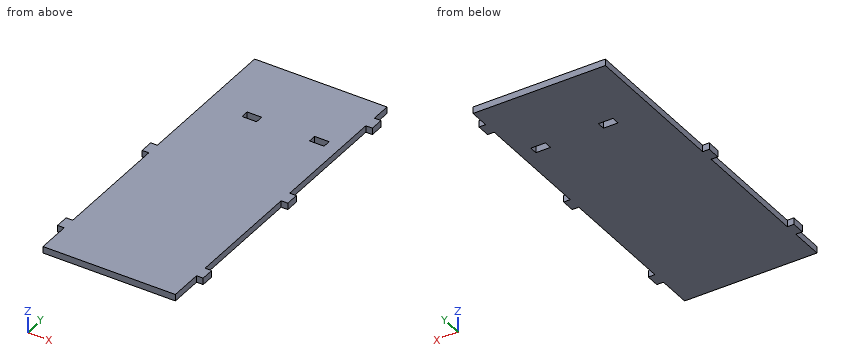
Autodesk Inventor part; units mm, degrees
ref_plane "YZ Plane" through (0, 0, 0) normal (1, 0, 0) x (0, 1, 0)
ref_plane "XZ Plane" through (0, 0, 0) normal (0, 1, 0) x (-1, 0, 0)
ref_plane "XY Plane" through (0, 0, 0) normal (0, 0, 1) x (1, 0, 0)
sketch "Sketch1" plane through (0, 0, 0) normal (0, 0, 1) x (1, 0, 0)
  line L0 (-100.6151, -124.6674) -> (-100.6151, 125.3326)
  line L1 (-41.6151, -124.6674) -> (-41.6151, 125.3326) construction
  line L2 (-0.6151, -124.6674) -> (-0.6151, 73.3335)
  line L3 (-0.6151, -124.6674) -> (-100.6151, -124.6674)
  line L4 (4.3849, 110.4326) -> (-0.6151, 110.4326)
  line L5 (4.3849, 100.3326) -> (4.3849, 110.4326)
  line L6 (-0.6151, 100.3326) -> (4.3849, 100.3326)
  line L7 (4.3849, -89.5674) -> (-0.6151, -89.5674)
  line L8 (4.3849, -99.6674) -> (4.3849, -89.5674)
  line L9 (-0.6151, -99.6674) -> (4.3849, -99.6674)
  line L10 (-100.6151, 10.4326) -> (-100.6151, 0.3326)
  line L11 (-100.6151, 0.3326) -> (-0.6151, 0.3326) construction
  line L12 (-0.6151, 0.3326) -> (4.3849, 0.3326)
  line L13 (-0.6151, 0.3326) -> (4.3849, 0.3326)
  line L14 (4.3849, 0.3326) -> (4.3849, 10.4326)
  line L15 (4.3849, 0.3326) -> (4.3849, 10.4326)
  line L16 (4.3849, 10.4326) -> (-0.6151, 10.4326)
  line L17 (4.3849, 10.4326) -> (-0.6151, 10.4326)
  line L18 (-0.6151, 73.3335) -> (-0.6151, 125.3326)
  line L19 (-0.6151, 125.3326) -> (-0.6151, 75.3326)
  line L20 (-0.6151, 75.3326) -> (-100.6151, 75.3326) construction
  line L21 (-105.6151, -99.6674) -> (-105.6151, -89.5674)
  line L22 (-105.6151, -89.5674) -> (-100.6151, -89.5674)
  line L23 (-100.6151, -99.6674) -> (-105.6151, -99.6674)
  line L24 (-105.6151, 10.4326) -> (-100.6151, 10.4326)
  line L25 (-105.6151, 0.3326) -> (-105.6151, 10.4326)
  line L26 (-100.6151, 0.3326) -> (-105.6151, 0.3326)
  line L27 (-100.6151, 125.3326) -> (-0.6151, 125.3326)
  line L28 (-0.6151, 125.3326) -> (-10.6151, 125.3326)
  line L29 (-0.6151, 76.5945) -> (-0.6151, 125.3326)
  line L30 (-100.6151, 125.3326) -> (-90.6151, 125.3326)
  line L31 (-100.6151, 76.6641) -> (-100.6151, 125.3326)
  line L32 (-82.6151, 75.3326) -> (17.3849, 75.3326) construction
  line L33 (-10.6151, 72.6641) -> (-10.6151, 66.6641)
  line L34 (-21.6151, 72.6641) -> (-21.6151, 66.6641)
  line L35 (-61.6151, 72.6641) -> (-61.6151, 66.6641)
  line L36 (-72.6151, 72.6641) -> (-72.6151, 66.6641)
  line L37 (-21.6151, 72.6641) -> (-61.6151, 72.6641) construction
  line L38 (-21.6151, 66.6641) -> (-61.6151, 66.6641) construction
  line L39 (-10.6151, 66.6641) -> (-21.6151, 66.6641)
  line L40 (-10.6151, 72.6641) -> (-21.6151, 72.6641)
  line L41 (-61.6151, 72.6641) -> (-72.6151, 72.6641)
  line L42 (-61.6151, 66.6641) -> (-72.6151, 66.6641)
  line L43 (-72.6151, 66.6641) -> (-100.6151, 66.6641) construction
  line L44 (-72.6151, 72.6641) -> (-100.6151, 72.6641) construction
  point P0 (0, 0)
  point P1 (4.3849, 105.3826)
  point P2 (-10.6151, 69.6641)
  point P3 (4.3849, -94.6174)
  point P4 (4.3849, 5.3826)
  point P5 (4.3849, 5.3826)
  point P6 (-105.6151, -94.6174)
  point P7 (-105.6151, 5.3826)
  dimension "d1" = 11
  dimension "d4" = 40
  dimension "d6" = 5
  dimension "d7" = 10
  dimension "d8" = 100
extrude "Extrusion1" add sketch "Sketch1" along normal blind 5
properties part number "Lifting Sections back"
The listing builds one solid part. Answer for the finished solid, in the listing's coordinates (mm). Give positions to 0.01 mm unless a question says otherwise; leave off trailing zeros. Order: outer loops, then holes, each group sorted by start corner. A loop starts at its lowest first (then second) coordinate and runs counter-clockwise, first axis right, second up. Notation, with made-up numbers: (67.25, 35) -> (111.25, 35) arc R30 cw to (111.25, 60) -> close; hole circle Ø2 at (87, 33). An arc over 180 degrees is marked (long way). Answer as a JSON object with one key per item and string values. Group by question number.
Item 1: The part is cut by section B-B on z = 2.3. Give the number of separate pieces and of enclosed holes in the cut face, and give its area (3 significant figures).
Item 2: Flat-ended cylindrical pins translate along their axes: pin 1 (1 mm diameter, centred on x = -79, y = -79.5, fed in from -Z); pin 2 (1.5 mm diameter, centred on y = 69, z = 3, fed in from -X); pin 3 (1.5 mm diameter, centred on x = 1, z = 2.5, fed in from -Y); pin 4 (2 mm diameter, centred on y = 90.5, z = 2, fed in from +X). Find the tip coordinate at first contact, or state that the pin passes through.
Item 3: Consider L1, parallel to Y at x = -0.5, z = 4.7; L2, parallel to Y at x = -18, z = 1.1; L3, parallel to X at y = 43, z = 1.25. Determine where each line is inside the solid, lowest interval first. Write a range as from..to.
Item 4: The part is cut by section A-A on x = -69. Write down the section's boundary in (y, z), and give its area (3 significant figures).
Item 5: The part is cut by section C-C on y = -60. Write down the section's boundary in (x, z).
Result set:
{
 "1": {"separate pieces": "1", "enclosed holes": "2", "area": "25,100 mm²"},
 "2": {"pin 1": "z = 0", "pin 2": "x = -100.62", "pin 3": "y = -99.67", "pin 4": "x = -0.62"},
 "3": {"L1": "-99.67..-89.57, 0.33..10.43, 100.33..110.43", "L2": "-124.67..66.66, 72.66..125.33", "L3": "-100.62..-0.62"},
 "4": {"outline": "(-124.67, 0) -> (66.66, 0) -> (66.66, 5) -> (-124.67, 5) -> close; (72.66, 0) -> (125.33, 0) -> (125.33, 5) -> (72.66, 5) -> close", "area": "1,220 mm²"},
 "5": {"outline": "(-100.62, 0) -> (-0.62, 0) -> (-0.62, 5) -> (-100.62, 5) -> close"}
}
